For this review, take the finished solid that the model builds, in its own axes (mm). Face numbers are marked on the shaded views. A direction names the side the tool comes from. Round coordinates to 2 decimals unless told otherwise and drop trailing zeros. Write each loop counter-clockwise with the first axis right and the second up, starting at its lowest first coordinate (ties: lowest second). Pieces come first, ordered by that corner, then holes. Notation, with made-up numbers: (82, 61.25) -> (96, 61.25) arc R33 cw to (96, 92.25) -> close; hole circle Ø6 at (-22, -1.5). An arc over 180 degrees is marked (long way). Write each question's results on one line, items separated by ' | '. Start each with the question number.
Item 1: Clearance check with flat-ended pins moving along their axes: pin 1 (2 mm diameter, centred on y = -84, z = 31, fed in from -X); pin 2 (6 mm diameter, centred on x = -47, y = -7.5, fed in from -Z); pin 3 (4 mm diameter, centred on x = -66.5, y = -49, fed in from +Z). State where each tip first meets the part, or that it passes through.
Item 2: Add section B-B (z = 0). State the section outline as (x, y) points (3 decimals), plus the area to 3 significant figures.
Item 3: To check wall thickness, follow line 1 along Y through (x, z) = (-51.5, 45) (3 decimals); line 2 along Z through (x, y) = (-61, -22). State the ranges of each line that lie inside material, in increasing order.
Item 4: Tool access review of the marked faces 1, 2 and 3: name each direction out of +Z, -Z, +X, -X, +Y, -Y from which nothing blocks a thin tool from reaching the whole face with its end or side.
Item 5: Add section A-A (z = -30.5). State the section outline as (x, y) points (3 decimals), plus the area to 3 significant figures.
Item 6: The part is to be moulded in two halves that separate along X. For the marked faces 4, 5 and 6, say which applies: +X half, -X half, draft (parallel to the pull), parting line (faces both ways), or undercut.
from build123d import *

# Parameters (mm, degrees)
F0_R     = 38.1
F0_R_2   = 34.925
F1_ANGLE = 90
F2_R     = 50.8
F2_R_2   = 34.925
F3_DEPTH = 9.525
F4_R     = 50.8
F4_R_2   = 34.925
F5_DEPTH = 9.525


with BuildPart() as f1:
    # F0 (on Front) → F1 (revolve)
    with BuildSketch(Plane.XZ):
        with Locations((-53.975, 0)):
            Circle(F0_R)
        with Locations((-53.975, 0)):
            Circle(F0_R_2, mode=Mode.SUBTRACT)
    revolve(axis=Axis((0, 0, 27.08186), (0, 0, 1)), revolution_arc=F1_ANGLE)

    # F2 (on face) → F3 (join)
    with BuildSketch(Plane.YZ):
        with Locations((-53.975, 0)):
            Circle(F2_R)
        with Locations((-53.975, 0)):
            Circle(F2_R_2, mode=Mode.SUBTRACT)
    extrude(amount=F3_DEPTH)

    # F4 (on face) → F5 (join)
    with BuildSketch(Plane(origin=(0, 0, 0), x_dir=(-1, 0, 0), z_dir=(0, 1, 0))):
        with Locations((53.975, 0)):
            Circle(F4_R)
        with Locations((53.975, 0)):
            Circle(F4_R_2, mode=Mode.SUBTRACT)
    extrude(amount=F5_DEPTH)


solid = f1.part
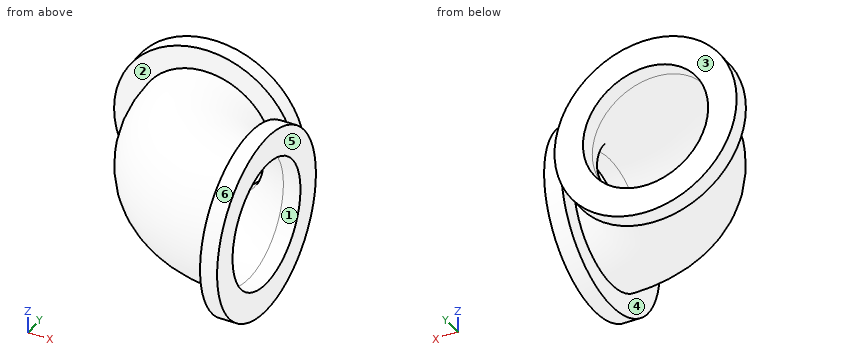
Responses:
1) pin 1: stops at x = 0 | pin 2: stops at z = -37.95 | pin 3: stops at z = 27.25
2) outline: (-104.775, 0) -> (-92.075, 0) arc R92.075 ccw to (0, -92.075) -> (0, -104.775) -> (9.525, -104.775) -> (9.525, -88.9) -> (0, -88.9) arc R88.9 cw to (-88.9, 0) -> (-88.9, 9.525) -> (-104.775, 9.525) -> close; (-19.05, 0) arc R19.05 ccw to (0, -19.05) -> (9.525, -19.05) -> (9.525, -3.175) -> (0, -3.175) -> (0, -15.875) arc R15.875 cw to (-15.875, 0) -> (-3.175, 0) -> (-3.175, 9.525) -> (-19.05, 9.525) -> close | area: 1,140 mm^2
3) line 1: y = 0 to 9.525 | line 2: z = -36.52 to -33.19, 33.19 to 36.52
4) face 1: +X | face 2: none | face 3: +Z, -Z, +X, -X, +Y
5) outline: (-94.6, 0) -> (-76.808, 0) arc R76.808 ccw to (0, -76.808) -> (0, -94.6) -> (9.525, -94.6) -> (9.525, -70.99) -> (0, -70.99) arc R70.99 cw to (-70.99, 0) -> (-70.99, 9.525) -> (-94.6, 9.525) -> close; (-36.96, 0) arc R36.96 ccw to (0, -36.96) -> (9.525, -36.96) -> (9.525, -13.35) -> (0, -13.35) -> (0, -31.142) arc R31.142 cw to (-31.142, 0) -> (-13.35, 0) -> (-13.35, 9.525) -> (-36.96, 9.525) -> close | area: 1,890 mm^2
6) face 4: undercut | face 5: +X half | face 6: draft
